```python
from build123d import *

# Parameters (mm, degrees)
F0_R     = 15
F1_DEPTH = 37.5
F2_R     = 2
F3_R     = 6
F4_DEPTH = 75.001


with BuildPart() as f1:
    # F0 (on Top) → F1 (new body, symmetric)
    with BuildSketch(Plane.XY):
        Circle(F0_R)
    extrude(amount=F1_DEPTH, both=True)

    # F2
    f2_edges = [f1.edges().sort_by_distance(p)[0] for p in [
        (-15, 0, 37.5),
        (-15, 0, -37.5),
    ]]
    fillet(f2_edges, radius=F2_R)

    # F3 (on face) → F4 (cut, through all)
    with BuildSketch(Plane.XY.offset(37.5)):
        Circle(F3_R)
    extrude(amount=-F4_DEPTH, mode=Mode.SUBTRACT)


solid = f1.part
```
Geometry: final body of the model. Coordinates: model frame, mm. Round coordinates to 2 decimals unless told otherwise and drop trailing zeros. Loops run counter-clockwise (first coordinate to the right, second up) from the corner with the lowest first, then second, coordinate; pieces in that order, holes last. Notation, with made-up numbers: (39, 32.25) -> (58, 32.25) arc R16 cw to (58, 54.25) -> close; hole circle Ø1 at (-12, -22). An arc over 180 degrees is marked (long way). Write each question's results on one line, items separated by ' | '.
Item 1: Cut plane C-C on z = -18.5. Return the cut outline in (x, y).
Answers below:
outline: circle Ø30 at (0, 0); hole circle Ø12 at (0, 0)
Item 2: Cut plane A-A on x = 0. Return the cut outline in (y, z).
Answers below:
outline: (-15, -35.5) arc R2 ccw to (-13, -37.5) -> (-6, -37.5) -> (-6, 37.5) -> (-13, 37.5) arc R2 ccw to (-15, 35.5) -> close; (6, -37.5) -> (13, -37.5) arc R2 ccw to (15, -35.5) -> (15, 35.5) arc R2 ccw to (13, 37.5) -> (6, 37.5) -> close
Item 3: Line query: probe 1 along Y at (x, z) = (0, -6); probe 2 along X at (y, z) = (3.5, 16); probe 3 along X at (y, z) = (-2.25, 22). Output: solid intervals per line, ascending. Write a range as [from, to].
Answers below:
probe 1: y = [-15, -6], [6, 15] | probe 2: x = [-14.59, -4.87], [4.87, 14.59] | probe 3: x = [-14.83, -5.56], [5.56, 14.83]
Item 4: Pin query (flat end, axial travel): pin 1 Ø6 at (x, z) = (-6.5, 26) entering from +Y; pin 2 Ø5 at (x, z) = (10.5, 9.5) entering from -Y; pin 3 Ø1 at (y, z) = (4, 26.5) entering from +X. Return the tip coordinate at first contact, or that it passes through.
Answers below:
pin 1: stops at y = 14.59 | pin 2: stops at y = -12.69 | pin 3: stops at x = 14.59
Item 5: Pull-direction query (Y, two-part tool) for faces 1 (the face through (6, -3, 37.5)), 2 (the face through (-14.985, 0.66, 0.497)), 3 (the face through (-6, 0, 1)); classes: pulls with the +Y half, pulls with the -Y half, needs draft (parallel to the pull), parting line crosses it, or undercut.
Answers below:
face 1: needs draft | face 2: parting line crosses it | face 3: undercut
